Read the model definition and answer for the solid it produces. Units are mm, in the model's axes. A direction names the side the tool comes from. Coordinates: 2 decimals unless noted, no trailing zeros. Loops run counter-clockwise (first coordinate to the right, second up) from the corner with the lowest first, then second, coordinate; pieces in that order, holes last. Notation, with made-up numbers: M 81,62 L 123,62 A13 cw 123,77 Z; hole C 33,-28 d3. An arc over 180 degrees is marked long. Use one line per item in the form item = value. Start each with the question number.
1. The part is cut by section B-B (x = 89.5). Give the vertices of the cut face in (y, z), plus the area to 3 significant figures.
2. For a pull along Z with two mould halves and no side action, classify faces 1 (the flat face through (45.69, 13.8, -83.18)), 2 (the flat face through (52, 14, 0)), 3 (the flat face through (47, 28, -42)) as released by +Z, released by -Z, zero draft, split by the parting line, or undercut.
3. Flat-ended cylindrical pins translate along their axes: pin 1 (1 mm diameter, centred on y = 4, z = -81.5, fed in from -X); pin 2 (4 mm diameter, centred on y = 10, z = -70.5, fed in from -X); pin 3 (1 mm diameter, centred on x = 28, y = 9.5, fed in from -Z); pin 4 (1 mm diameter, centred on x = 23, y = 12, fed in from +Z). Find the tip coordinate at first contact, or state that the pin passes through.
4. A tool of negligible diameter and unlimited length cuts with its end or side. For faces 4 (the flat face through (105.76, 14, -33)), 5 (the flat face through (73, 14, -66.506)), from which of +Z, -Z, +X, -X, +Y, -Y can it reach the whole face along a straight path? Write none if from no direction.
5. Find the intervals of material crossed by probe 1 along Z at (x, y) = (87, 22); probe 2 along Z at (x, y) = (26, 24.75); probe 3 along X at (y, z) = (12, -78), in increasing order. Write a range as [from, to].
6. The part is cut by section A-A (z = -44). Give the vertices of the cut face in (x, y), plus the area to 3 significant figures.
from build123d import *

# Parameters (mm, degrees)
BOSS_EXTRUDE1_DEPTH = 28


with BuildPart() as part:
    # Sketch1 → Boss-Extrude1 (new body)
    with BuildSketch(Plane(origin=(0, 0, 0), x_dir=(1, 0, 0), z_dir=(0, 1, 0))):
        with BuildLine():
            Line((0, 0), (105.760379504, 0))
            Line((105.760379504, 0), (105.760379504, 66.505760117))
            Line((105.760379504, 66.505760117), (39.146479939, 66.505760117))
            Line((39.146479939, 66.505760117), (52.415736455, 100.323934711))
            add(Edge.make_bspline(
                [(52.415736455, 100.323934711), (50.07713871, 103.942471785), (41.897556232, 105.536469955), (34.280133355, 99.294275572), (32.228567822, 94.566792302), (30.972636221, 92.447002695)],
                knots=[0, 0, 0, 0, 0.447115865, 0.733607522, 1, 1, 1, 1], degree=3))
            Line((30.972636221, 92.447002695), (-6.571045616, 13.050137499))
            add(Edge.make_bspline(
                [(-6.571045616, 13.050137499), (-10.402799403, 7.920582359), (-5.185472177, 1.285466499), (0, 0)],
                knots=[0, 0, 0, 0, 1, 1, 1, 1], degree=3))
        make_face()
    extrude(amount=BOSS_EXTRUDE1_DEPTH)


solid = part.part
Computed values:
q1.outline = M 0,-66.51 L 28,-66.51 L 28,0 L 0,0 Z
q1.area = 1,860 mm²
q2.face_1 = undercut
q2.face_2 = released by +Z
q2.face_3 = zero draft
q3.pin_1 = 25.56
q3.pin_2 = 19.65
q3.pin_3 = -87.22
q3.pin_4 = 0
q4.face_4 = +Z, -Z, +X, +Y, -Y
q4.face_5 = +X, +Y, -Y
q5.probe_1 = [-66.51, 0]
q5.probe_2 = [-81.93, 0]
q5.probe_3 = [24.14, 43.66]
q6.outline = M 8.06,0 L 105.76,0 L 105.76,28 L 8.06,28 Z
q6.area = 2,740 mm²
